Geometry: final body of the model. Coordinates: model frame, mm. Face numbers are marked on the shaded views. A direction names the side the tool comes from. Coordinates: 2 decimals unless noted, no trailing zeros. Write each loop counter-clockwise with the first axis right and the second up, starting at its lowest first coordinate (ties: lowest second). Pieces come first, ordered by that corner, then holes.
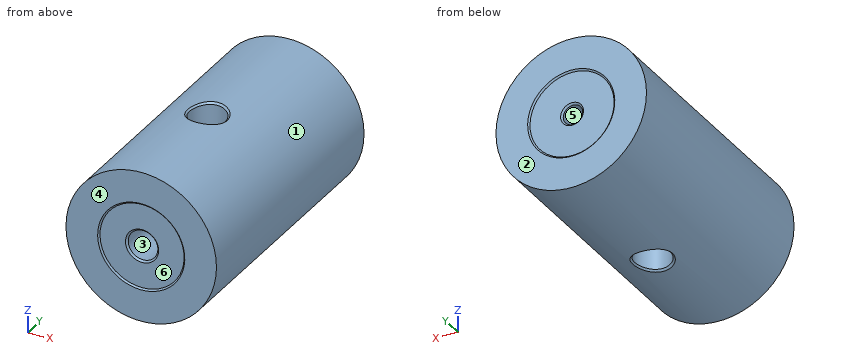
Autodesk Inventor part; units mm, degrees
ref_plane "YZ Plane" through (0, 0, 0) normal (1, 0, 0) x (0, 1, 0)
ref_plane "XZ Plane" through (0, 0, 0) normal (0, 1, 0) x (-1, 0, 0)
ref_plane "XY Plane" through (0, 0, 0) normal (0, 0, 1) x (1, 0, 0)
sketch "Sketch1" plane through (0, 0, 0) normal (0, 1, 0) x (-1, 0, 0)
  circle A0 centre (0, 0) radius 12.5
  dimension "d0" = 25
extrude "Extrusion1" add sketch "Sketch1" along normal blind 44.6
hole "ReliefTop" at (0, 44.6, 0) direction (0, -1, 0) diameter 13.97 depth 0.254 countersink diameter 14.478 countersink angle 90
hole "ReliefBottom" at (0, 0, 0) direction (0, 1, 0) diameter 13.97 depth 0.254 countersink diameter 14.478 countersink angle 90
hole "MountBottomM6" at (0, 0.254, 0) direction (0, 1, 0) diameter 4.917 depth 7.366 tip angle 118 countersink diameter 5.508 countersink angle 90
hole "MountTopM4" at (0, 44.346, 0) direction (0, -1, 0) diameter 3.242 depth 14.478 tip angle 118 countersink diameter 3.808 countersink angle 90
sketch "Sketch2" plane through (0, 0, 0) normal (0, 0, 1) x (1, 0, 0)
  circle A0 centre (0, 20) radius 3
  line L0 (-12.5, 0) -> (12.5, 0)
  line L1 (0, -4.6) -> (0, 27.6)
  point P0 (0, 0)
  dimension "d49" = 6
  dimension "d50" = 20
extrude "Extrusion2" cut sketch "Sketch2" along normal through all both and the other way through all
chamfer "Chamfer1" distance 0.313 angle 45 2 edges at (-3, 19.9998, 12.1347) (-3, 19.9998, -12.1347)
equation "\"d1\" = height"
equation "\"d5\" = reliefMinor"
equation "\"d7\" = reliefMajor"
equation "\"d10\" = reliefDepth"
equation "\"d14\" = reliefMinor"
equation "\"d16\" = reliefMajor"
equation "\"d19\" = reliefDepth"
equation "\"d25\" = chamferM6"
equation "\"d28\" = depthM6"
equation "\"d40\" = chamferM4"
equation "\"d43\" = depthM4"
equation "\"reliefDepth\" = 0.254"
equation "\"reliefMinor\" = 13.97"
equation "\"reliefMajor\" = 14.478"
equation "\"chamferM6\" = 5.508"
equation "\"chamferM4\" = 3.808"
equation "\"depthM6\" = 7.366"
equation "\"depthM4\" = 14.478"
equation "\"height\" = 44.6"
properties part number "PLS-P642H0446A00_M" material "Stainless Steel"
Item 1: Section B-B, the plane y = 14. Output: boundary loops of the cut face in (x, z).
Derived:
outline: circle Ø25 at (0, 0)
Item 2: Set-up query: the marked faces 4, 5 and 6. Return all of +Z, -Z, +X, -X, +Y, -Y with unobstructed straight access to the full face (end or side cutting, diameter ignored); none if empty.
Derived:
face 4: +Z, -Z, +X, -X, -Y
face 5: +Y
face 6: -Y
Item 3: Pin query (flat end, axial travel): pin 1 (3 mm diameter, centred on x = 8, z = -9, fed in from -Y); pin 2 (1 mm diameter, centred on x = 7.5, y = 16.5, fed in from -Z); pin 3 (4 mm diameter, centred on x = -3.5, z = 0, fed in from +Y); pin 4 (8 mm diameter, centred on y = 40, z = 5.5, fed in from +X). Return the tip coordinate at first contact, or that it passes through.
Derived:
pin 1: stops at y = 0
pin 2: stops at z = -10.36
pin 3: stops at y = 44.35
pin 4: stops at x = 12.41
Item 4: Section C-C, the plane z = 7.75. Output: boundary loops of the cut face in (x, y), plus the area to 3 significant figures.
Derived:
outline: (-9.81, 0) - (9.81, 0) - (9.81, 44.6) - (-9.81, 44.6) - close; hole circle Ø6 at (0, 20)
area: 847 mm2
Item 5: Pull-direction query (Z, two-part tool) for the marked faces 1, 2 and 3; classes: released by +Z, released by -Z, zero draft, split by the parting line, or undercut.
Derived:
face 1: split by the parting line
face 2: zero draft
face 3: undercut
Item 6: Material intervals for probe 1 along Z at (x, y) = (0, 2); probe 2 along Y at (x, z) = (0.25, 7.25); probe 3 along Z at (x, y) = (0, 33.25), sorted ascending.
Derived:
probe 1: z = -12.5 to -2.46, 2.46 to 12.5
probe 2: y = 0 to 17.01, 22.99 to 44.6
probe 3: z = -12.5 to -1.62, 1.62 to 12.5
Item 7: Section A-A, the plane y = 3.5. Output: boundary loops of the cut face in (x, z), plus the area to 3 significant figures.
Derived:
outline: circle Ø25 at (0, 0); hole circle Ø4.92 at (0, 0)
area: 472 mm2
Item 8: Section D-D, the plane x = 8. Output: boundary loops of the cut face in (y, z).
Derived:
outline: (0, -9.6) - (44.6, -9.6) - (44.6, 9.6) - (0, 9.6) - close
